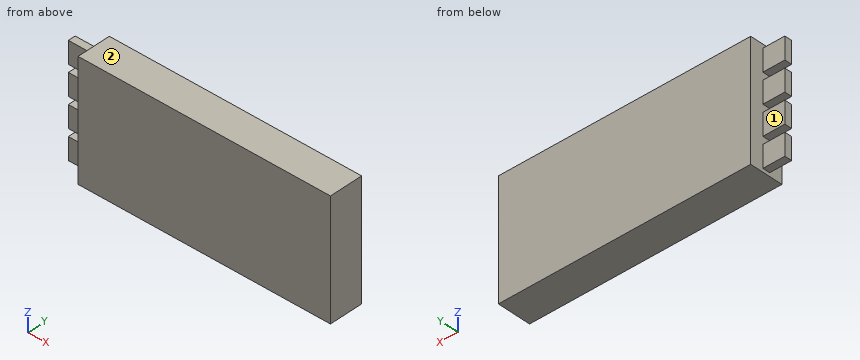
```python
from build123d import *

# Parameters (mm, degrees)
SKETCH1_W           = 172.5
SKETCH1_H           = 80
BOSS_EXTRUDE1_DEPTH = 23
SKETCH2_W           = 15
SKETCH2_H           = 5
BOSS_EXTRUDE2_DEPTH = 15


with BuildPart() as part:
    # Sketch1 → Boss-Extrude1 (new body)
    with BuildSketch(Plane(origin=(0, 0, 0), x_dir=(1, 0, 0), z_dir=(0, 1, 0))):
        Rectangle(SKETCH1_W, SKETCH1_H)
    extrude(amount=BOSS_EXTRUDE1_DEPTH)

    # Sketch2 → Boss-Extrude2 (add)
    with BuildSketch(Plane.ZY.offset(86.25)):
        with Locations((9.965110339, 11.5)):
            Rectangle(SKETCH2_W, SKETCH2_H)
        with Locations((30, 11.5)):
            Rectangle(SKETCH2_W, SKETCH2_H)
        with Locations((-10.069779322, 11.5)):
            Rectangle(SKETCH2_W, SKETCH2_H)
        with Locations((-30.104668983, 11.5)):
            Rectangle(SKETCH2_W, SKETCH2_H)
    extrude(amount=BOSS_EXTRUDE2_DEPTH)


solid = part.part
```
Source: CAD feature listing. Evaluate the final solid. Frame: model axes, mm. Face numbers are marked on the shaded views. A direction names the side the tool comes from. Give positions to 0.01 mm unless a question says otherwise; leave off trailing zeros. Loops run counter-clockwise (first coordinate to the right, second up) from the corner with the lowest first, then second, coordinate; pieces in that order, holes last. Notation, with made-up numbers: (-36.75, 42) -> (-29.75, 42) arc R3 cw to (-29.75, 46) -> close; hole circle Ø7 at (9, 37). An arc over 180 degrees is marked (long way). Use a Markdown table: item, result. Add a question column.
(1) Section query B-B (y = 12.25). Output: boundary loops of the cut face in (x, z), then the cut area to 3 significant figures.
(2) First-contact query: pin 1 Ø16.5 at (x, z) = (-96, -31) entering from +Y; pin 2 Ø4.5 at (x, z) = (-95.5, -11.5) entering from -Y; pin 3 Ø4 at (x, y) = (-91, 11) entering from +Z. Flat tips, straight axial feed; report the tip coordinate or a pass-through.
(3) Access query for the marked faces 1 and 2. Directions: +Z, -Z, +X, -X, +Y, -Y. A direction counts if a zero-diameter tool reaches every point of the face in a straight line with its end or side. Return the directions, or none.
(4) Section query A-A (z = 15). Output: boundary loops of the cut face in (x, y), then the cut area to 3 significant figures.
(5) Ray query, line 1 (X direction, y = 3.5, z = -16); line 2 (Y direction, x = -86.5, z = 8). Return the intervals inside material, ascending.
Checked values:
| question | item | result |
|---|---|---|
| 1 | outline | (-101.25, -37.6) -> (-86.25, -37.6) -> (-86.25, -40) -> (86.25, -40) -> (86.25, 40) -> (-86.25, 40) -> (-86.25, 37.5) -> (-101.25, 37.5) -> (-101.25, 22.5) -> (-86.25, 22.5) -> (-86.25, 17.47) -> (-101.25, 17.47) -> (-101.25, 2.47) -> (-86.25, 2.47) -> (-86.25, -2.57) -> (-101.25, -2.57) -> (-101.25, -17.57) -> (-86.25, -17.57) -> (-86.25, -22.6) -> (-101.25, -22.6) -> close |
| 1 | area | 14,700 mm^2 |
| 2 | pin 1 | y = 14 |
| 2 | pin 2 | y = 9 |
| 2 | pin 3 | z = 37.5 |
| 3 | face 1 | +Z, -Z, -X, +Y |
| 3 | face 2 | +Z, +X, -X, +Y, -Y |
| 4 | outline | (-101.25, 9) -> (-86.25, 9) -> (-86.25, 0) -> (86.25, 0) -> (86.25, 23) -> (-86.25, 23) -> (-86.25, 14) -> (-101.25, 14) -> close |
| 4 | area | 4,040 mm^2 |
| 5 | line 1 | -86.25 to 86.25 |
| 5 | line 2 | 9 to 14 |
